from build123d import *

# Parameters (mm, degrees)
F0_W     = 61.931412667
F0_H     = 55.6655190885
F0_H_2   = 49.976002425
F0_W_2   = 54.4153526425
F1_DEPTH = 25.4
F2_W     = 29.6337604523
F2_H     = 28.9934612811
F2_W_2   = 27.0190127194
F3_DEPTH = 25.4
F5_DEPTH = 25.4


with BuildPart() as f1:
    # F0 (on Top) → F1 (new body)
    with BuildSketch(Plane.XY):
        with Locations((30.9657063335, 27.8327595443)):
            Rectangle(F0_W, F0_H)
        with Locations((30.9657063335, -24.9880012125)):
            Rectangle(F0_W, F0_H_2)
        with Locations((-27.2076763213, -24.9880012125)):
            Rectangle(F0_W_2, F0_H_2)
        with Locations((-27.2076763213, 27.8327595443)):
            Rectangle(F0_W_2, F0_H)
    extrude(amount=F1_DEPTH)

    # F2 (on Front) → F3 (join)
    with BuildSketch(Plane.XZ):
        Polygon((0, 0), (0, 8.6490437388), (-29.6337604523, 8.6490437388), (-29.6337604523, -16.8678652386), align=None)
        with Locations((-14.8168802261, 23.1457743794)):
            Rectangle(F2_W, F2_H)
        with Locations((13.5095063597, 23.1457743794)):
            Rectangle(F2_W_2, F2_H)
        Polygon((27.0190127194, 8.6490437388), (0, 8.6490437388), (0, 0), (0, -22.8965952992), (27.0190127194, -22.8965952992), align=None)
        Polygon((0, -22.8965952992), (0, 0), (-29.6337604523, -16.8678652386), (-29.6337604523, -22.8965952992), align=None)
        Polygon((-29.6337604523, -22.8965952992), (-29.6337604523, -16.8678652386), (-212.6657664776, -121.0517138243), (0, -22.8965952992), align=None)
    extrude(amount=F3_DEPTH)

    # F4 (on Right) → F5 (join)
    with BuildSketch(Plane.YZ):
        Polygon((0, -18.9130362123), (0, 0), (-479.4011116028, 194.1131353378), align=None)
    extrude(amount=F5_DEPTH)


solid = f1.part
Part model, mm, in its own coordinate system. A direction names the side the tool comes from. Coordinates: 2 decimals unless noted, no trailing zeros. Loops run counter-clockwise (first coordinate to the right, second up) from the corner with the lowest first, then second, coordinate; pieces in that order, holes last. Notation, with made-up numbers: M 53,43.25 L 71,43.25 A17 ccw 71,54.25 Z; hole C 15,-35.5 d3. An arc over 180 degrees is marked long. Use a Markdown table: item, result. Add a question column.
Q1. Cut at B-B (y = -17). Write the cut outline in (x, z).
Q2. Cut at A-A (x = 14). Write the cut outline in (y, z), and give its area (3 significant figures).
Q3. Pin check, flat tips, straight feed: P1, Ø20.5, axis at x = 9, y = -16.5, coming from the -Z side; P2, Ø7.5, axis at x = 6.5, y = -13.5, coming from the +Z side; P3, Ø3.5, axis at y = -18.5, z = 31.5, coming from the +X side; P4, Ø8, axis at y = -30.5, z = -73.5, coming from the +X side. Stop position of each tip, or through.
Q4. Cut at D-D (y = -290.5). Write the cut outline in (x, z).
Q5. Which spindle directions (+Z, -Z, +X, -X, +Y, -Y) get a long thin tool onto all of the face, cutting with end or side? Do faces 1 (the flat face through (0, -154, 57)), 2 (the flat face through (13, -13, -22.897)), 3 (the flat face through (-2, -25.4, 32)), 4 (the flat face through (-58, 0, -38)), 5 (the flat face through (27.019, -13, 31)). Say none if no direction does.
Q6. Probe L1, parallel to Z at x = -42, y = 16.5; L2, parallel to X at y = 22.5, z = 14; L3, parallel to Z at x = -157.5, y = -3. List the from-to ranges inside material, lowest first.
Q7. Cut at C-C (z = 134). Write the cut outline in (x, y), and give its area (3 significant figures).
Worked out:
| question | item | result |
|---|---|---|
| 1 | outline | M -212.67,-121.05 L 0,-22.9 L 27.02,-22.9 L 27.02,0 L 61.93,0 L 61.93,25.4 L 27.02,25.4 L 27.02,37.64 L -29.63,37.64 L -29.63,25.4 L -54.42,25.4 L -54.42,0 L -29.63,0 L -29.63,-16.87 Z |
| 2 | outline | M -479.4,194.11 L -49.98,3.29 L -49.98,0 L -42.56,0 L -25.4,-7.63 L -25.4,-22.9 L 0,-22.9 L 0,0 L 55.67,0 L 55.67,25.4 L 0,25.4 L 0,37.64 L -25.4,37.64 L -25.4,25.4 L -49.98,25.4 L -49.98,20.24 Z |
| 2 | area | 7,280 mm2 |
| 3 | P1 | stops at z = -23.47 |
| 3 | P2 | stops at z = 37.64 |
| 3 | P3 | stops at x = 27.02 |
| 3 | P4 | passes through |
| 4 | outline | M 0,110.17 L 25.4,110.17 L 25.4,117.63 L 0,117.63 Z |
| 5 | face 1 | +Z, -Z, -X, -Y |
| 5 | face 2 | -Z, +X, +Y, -Y |
| 5 | face 3 | +Z, +X, -X |
| 5 | face 4 | -Z, +X, -X, +Y |
| 5 | face 5 | +Z, +X, +Y, -Y |
| 6 | L1 | z = 0 to 25.4 |
| 6 | L2 | x = -54.42 to 61.93 |
| 6 | L3 | z = -95.59 to -89.65 |
| 7 | outline | M 0,-344.12 L 25.4,-344.12 L 25.4,-330.94 L 0,-330.94 Z |
| 7 | area | 335 mm2 |
